```python
from build123d import *

# Parameters (mm, degrees)
F1_DEPTH = 3.175
F2_W     = 15.875
F2_H     = 92.075
F3_DEPTH = 1.5875
F4_W     = 3.175
F4_H     = 31.75
F5_DEPTH = 3.175
F6_W     = 4.7625
F6_H     = 1.5875
F7_DEPTH = 4.7635
F8_W     = 4.7625
F8_H     = 1.5875
F9_DEPTH = 4.7635


with BuildPart() as f1:
    # F0 (on Top) → F1 (new body)
    with BuildSketch(Plane.XY):
        Polygon((7.9375, 49.2125), (-7.9375, 49.2125), (-7.9375, 26.19375), (-12.7, 26.19375), (-12.7, -18.25625), (-7.9375, -18.25625), (-7.9375, -42.8625), (7.9375, -42.8625), (7.9375, -18.25625), (12.7, -18.25625), (12.7, 26.19375), (7.9375, 26.19375), align=None)
    extrude(amount=F1_DEPTH)

    # F2 (on face) → F3 (join)
    with BuildSketch(Plane(origin=(0, 0, 0), x_dir=(1, 0, 0), z_dir=(0, 0, -1))):
        with Locations((0, -3.175)):
            Rectangle(F2_W, F2_H)
    extrude(amount=F3_DEPTH)

    # F4 (on face) → F5 (cut)
    with BuildSketch(Plane.XY.offset(3.175)):
        with Locations((0, 3.96875)):
            Rectangle(F4_W, F4_H)
    extrude(amount=-F5_DEPTH, mode=Mode.SUBTRACT)

    # F6 (on face) → F7 (cut, through all)
    with BuildSketch(Plane.XY.offset(3.175)):
        with Locations((0, -42.06875)):
            Rectangle(F6_W, F6_H)
    extrude(amount=-F7_DEPTH, mode=Mode.SUBTRACT)

    # F8 (on face) → F9 (cut, through all)
    with BuildSketch(Plane.XY.offset(3.175)):
        with Locations((0, 44.053125)):
            Rectangle(F8_W, F8_H)
    extrude(amount=-F9_DEPTH, mode=Mode.SUBTRACT)


solid = f1.part
```
Geometry: final body of the model. Coordinates: model frame, mm. A direction names the side the tool comes from. Round coordinates to 2 decimals unless told otherwise and drop trailing zeros. Write each loop counter-clockwise with the first axis right and the second up, starting at its lowest first coordinate (ties: lowest second). Pieces come first, ordered by that corner, then holes. Notation, with made-up numbers: (-5, 22.25) -> (49, 22.25) arc R26 cw to (49, 53.25) -> close; hole circle Ø2 at (10, -16). An arc over 180 degrees is marked (long way). Return JSON: item names as keys, results as strings.
Q1. Set-up query: faces 1 (the flat face through (0, 44.847, 1)), 2 (the flat face through (-1.588, 4, 2)), 3 (the flat face through (-10, -18.256, 2)). Return all of +Z, -Z, +X, -X, +Y, -Y with unobstructed straight access to the full face (end or side cutting, diameter ignored); none if empty.
From the geometry:
{"face 1": "+Z, -Z", "face 2": "+Z", "face 3": "+Z, -Z, -X, -Y"}
Q2. First-contact query: pin 1 Ø1.3 at (y, z) = (-42, 1) entering from +X; pin 2 Ø1 at (x, z) = (-9.5, 1.5) entering from +Y; pin 3 Ø2.5 at (x, z) = (-0.5, -0.5) entering from -Y (3 decimals). Flat tips, straight axial feed; report the tip coordinate or a pass-through.
From the geometry:
{"pin 1": "x = 7.94", "pin 2": "y = 26.19", "pin 3": "y = -41.275"}
Q3. Mould query, pull axis Y, two halves, no side actions, for faces 4 (the flat face through (10, 26.194, 2)), 5 (the flat face through (0, -11.906, 2)), 6 (the flat face through (2.381, -42, 1)). Classes: +Y half, -Y half, draft (parallel to the pull), parting line (faces both ways), or undercut.
From the geometry:
{"face 4": "+Y half", "face 5": "undercut", "face 6": "draft"}
Q4. Section D-D on y = 23. Return the cut outline in (x, z) (1 decimal), and give its area (3 significant figures).
From the geometry:
{"outline": "(-12.7, 0) -> (-7.9, 0) -> (-7.9, -1.6) -> (7.9, -1.6) -> (7.9, 0) -> (12.7, 0) -> (12.7, 3.2) -> (-12.7, 3.2) -> close", "area": "106 mm2"}
Q5. Ray query, line 1 (Y direction, x = 0.5, z = 1.3) (1 decimal); line 2 (Y direction, x = 1, z = -1) (1 decimal); line 3 (X direction, y = 19, z = 1.25). Return the intervals inside material, ascending.
From the geometry:
{"line 1": "-41.3 to -11.9, 19.8 to 43.3, 44.8 to 49.2", "line 2": "-41.3 to 43.3, 44.8 to 49.2", "line 3": "-12.7 to -1.59, 1.59 to 12.7"}
Q6. Section C-C on y = -3. Return the cut outline in (x, z) (1 decimal).
From the geometry:
{"outline": "(-12.7, 0) -> (-7.9, 0) -> (-7.9, -1.6) -> (7.9, -1.6) -> (7.9, 0) -> (12.7, 0) -> (12.7, 3.2) -> (1.6, 3.2) -> (1.6, 0) -> (-1.6, 0) -> (-1.6, 3.2) -> (-12.7, 3.2) -> close"}
Q7. Section B-B on z = 1. Return the cut outline in (x, y) (1 decimal).
From the geometry:
{"outline": "(-12.7, -18.3) -> (-7.9, -18.3) -> (-7.9, -42.9) -> (-2.4, -42.9) -> (-2.4, -41.3) -> (2.4, -41.3) -> (2.4, -42.9) -> (7.9, -42.9) -> (7.9, -18.3) -> (12.7, -18.3) -> (12.7, 26.2) -> (7.9, 26.2) -> (7.9, 49.2) -> (-7.9, 49.2) -> (-7.9, 26.2) -> (-12.7, 26.2) -> close; hole (-2.4, 43.3) -> (2.4, 43.3) -> (2.4, 44.8) -> (-2.4, 44.8) -> close; hole (-1.6, -11.9) -> (1.6, -11.9) -> (1.6, 19.8) -> (-1.6, 19.8) -> close"}
Q8. Section A-A on x = 0. Return the cut outline in (y, z) (1 decimal), and give its area (3 significant figures).
From the geometry:
{"outline": "(-41.3, -1.6) -> (43.3, -1.6) -> (43.3, 3.2) -> (19.8, 3.2) -> (19.8, 0) -> (-11.9, 0) -> (-11.9, 3.2) -> (-41.3, 3.2) -> close; (44.8, -1.6) -> (49.2, -1.6) -> (49.2, 3.2) -> (44.8, 3.2) -> close", "area": "323 mm2"}
